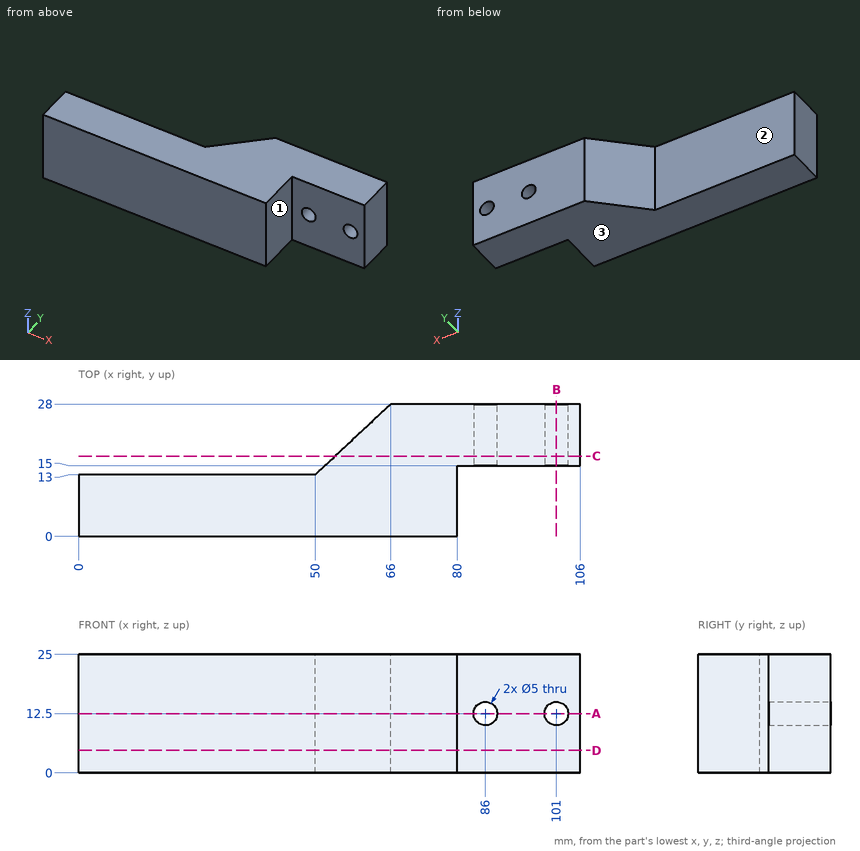
Geometry check sheet. Reference: drawing and pictorial views, mm from the part's lowest x, y, z. A direction names the side the tool comes from. Coordinates: 2 decimals unless noted, no trailing zeros. Order: outer loops, then holes, each group sorted by start corner. A loop starts at its lowest first (then second) coordinate and runs counter-clockwise, first axis right, second up.
Item 1: Section check A-A (z = 12.5). Enter the section's corners in (x, y).
Item 2: Section check D-D (z = 4.75). Enter the section's corners in (x, y).
Item 3: Section check B-B (x = 101). Enter the section's corners in (y, z).
Item 4: Depth check by flat-ended pin: pin 1 (12.5 mm diameter, centred on x = 29, z = 12.5, fed in from +Y); pin 2 (4 mm diameter, centred on x = 93, z = 4, fed in from -Y); pin 3 (8 mm diameter, centred on y = 5, z = 22.5, fed in from +X). Enter the tip coordinate at first touch or a pass-through.
Item 5: Tool access check on the marked faces 1, 2 and 3. Record the directions out of +Z, -Z, +X, -X, +Y, -Y that give a thin tool (end or side, any length) a straight path to the whole face; none if there is none.
Item 6: Section check C-C (y = 17). Enter the section's corners in (x, z).
Item 7: Scan lines: line 1 along Z through (x, y) = (101, 25.5); line 2 along X through (y, z) = (24.5, 14.5); line 3 along X through (y, z) = (17.75, 13.5). Record each from-to range of solid material in increasing order.
Check sheet entries:
1. outline: (0, 0) - (80, 0) - (80, 15) - (83.5, 15) - (83.5, 28) - (66, 28) - (50, 13) - (0, 13) - close; (88.5, 15) - (98.5, 15) - (98.5, 28) - (88.5, 28) - close; (103.5, 15) - (106, 15) - (106, 28) - (103.5, 28) - close
2. outline: (0, 0) - (80, 0) - (80, 15) - (106, 15) - (106, 28) - (66, 28) - (50, 13) - (0, 13) - close
3. outline: (15, 0) - (28, 0) - (28, 10) - (15, 10) - close; (15, 15) - (28, 15) - (28, 25) - (15, 25) - close
4. pin 1: stops at y = 13
4. pin 2: stops at y = 15
4. pin 3: stops at x = 80
5. face 1: +Z, -Z, +X, -Y
5. face 2: +Z, -Z, -X, +Y
5. face 3: -Z, +X, -X, +Y, -Y
6. outline: (54.27, 0) - (106, 0) - (106, 25) - (54.27, 25) - close; hole circle Ø5 at (86, 12.5); hole circle Ø5 at (101, 12.5)
7. line 1: z = 0 to 10, 15 to 25
7. line 2: x = 62.27 to 84.5, 87.5 to 99.5, 102.5 to 106
7. line 3: x = 55.07 to 83.71, 88.29 to 98.71, 103.29 to 106
